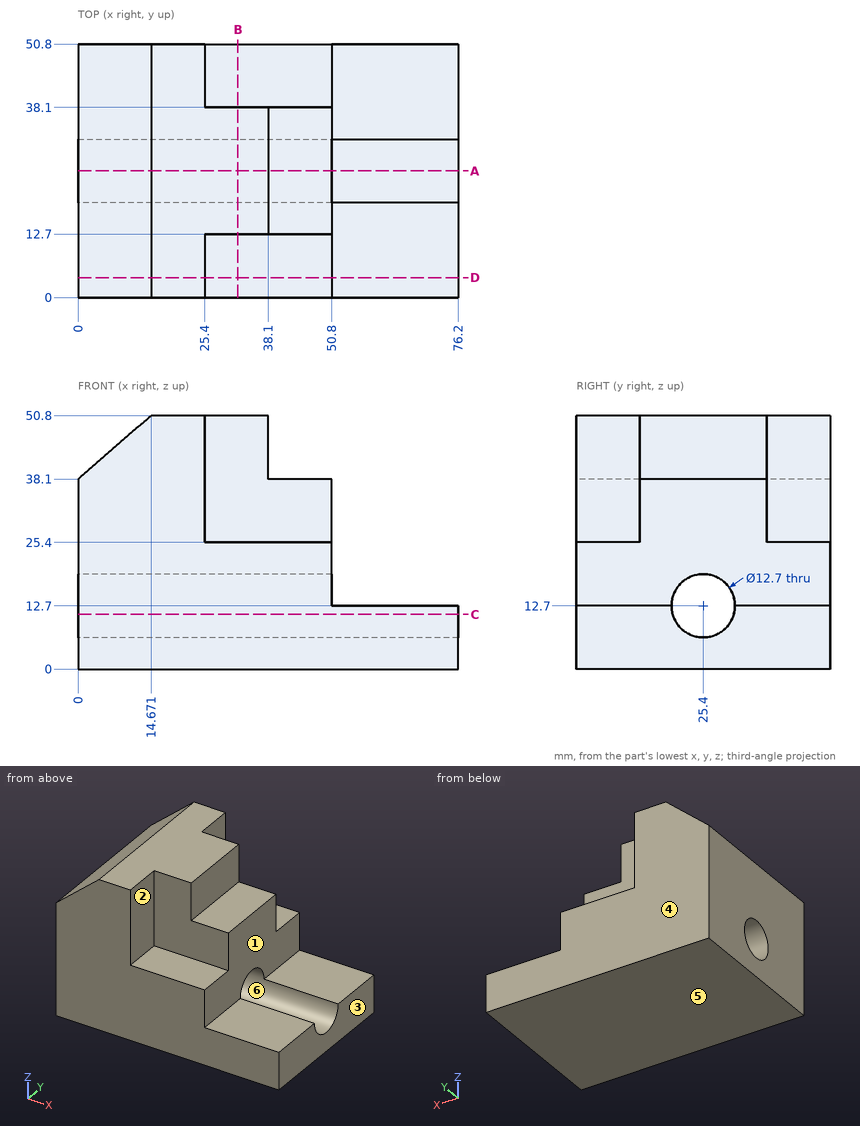
Job drawing, mm, ordinate dimensions from the low corner. One solid piece. A direction names the side the tool comes from. Give positions to 0.01 mm unless a question says otherwise; leave off trailing zeros. Write each loop counter-clockwise with the first axis right and the second up, starting at its lowest first coordinate (ties: lowest second). Pieces come first, ordered by that corner, then holes. Notation, with made-up numbers: M 77.5,68 L 118.5,68 A9 ccw 118.5,73 Z; hole C 12.5,-17 d10. An arc over 180 degrees is marked long. Put each result on its own line as item: value. Start each with the question number.
(1) Probe L1, parallel to Z at x = 47, y = 25; L2, parallel to Z at x = 38, y = 25; L3, parallel to X at y = 32.5, z = 21. List the from-to ranges inside material, lowest first.
(2) Flat gauge pins, fed straight in: pin 1 Ø4 at (y, z) = (4, 36) entering from +X; pin 2 Ø12.5 at (x, z) = (42.5, 41.5) entering from +Y; pin 3 Ø21 at (x, y) = (69, 10) entering from +Z. Where does each tip first touch, or does it go through?
(3) Mould opens along Y. For the marked faces 4, 5 and 6 say: +Y half, -Y half, draft (parallel to the pull), parting line (faces both ways), or undercut.
(4) Band-saw the part on A-A, the plane y = 25.4. Write the cut outline in (x, z).
(5) Band-saw the part on B-B, the plane x = 32. Write the cut outline in (y, z), and give its area (3 significant figures).
(6) Which spindle directions (+Z, -Z, +X, -X, +Y, -Y) get a long thin tool onto all of the face, cutting with end or side? Do the marked faces 1, 2 and 3. Say none if no direction does.
(7) Band-saw the part on D-D, the plane y = 4. Write the cut outline in (x, z).
(8) Band-saw the part on C-C, the plane z = 11. Write the cut outline in (x, y), and give its area (3 significant figures).
Response values:
1. L1: z = 0 to 6.36, 19.04 to 38.1
1. L2: z = 0 to 6.36, 19.04 to 50.8
1. L3: x = 0 to 50.8
2. pin 1: stops at x = 25.4
2. pin 2: stops at y = 38.1
2. pin 3: stops at z = 12.7
3. face 4: +Y half
3. face 5: draft
3. face 6: undercut
4. outline: M 0,0 L 76.2,0 L 76.2,6.35 L 0,6.35 Z; M 0,19.05 L 50.8,19.05 L 50.8,38.1 L 38.1,38.1 L 38.1,50.8 L 14.67,50.8 L 0,38.1 Z
5. outline: M 0,0 L 50.8,0 L 50.8,25.4 L 38.1,25.4 L 38.1,50.8 L 12.7,50.8 L 12.7,25.4 L 0,25.4 Z; hole C 25.4,12.7 d12.7
5. area: 1,810 mm2
6. face 1: +Z, +X, +Y, -Y
6. face 2: +Z, +X, -Y
6. face 3: +Z, -Z, +X, +Y, -Y
7. outline: M 0,0 L 76.2,0 L 76.2,12.7 L 50.8,12.7 L 50.8,25.4 L 25.4,25.4 L 25.4,50.8 L 14.67,50.8 L 0,38.1 Z
8. outline: M 0,0 L 76.2,0 L 76.2,19.28 L 0,19.28 Z; M 0,31.52 L 76.2,31.52 L 76.2,50.8 L 0,50.8 Z
8. area: 2,940 mm2
